Part model, mm, in its own coordinate system. Round coordinates to 2 decimals unless told otherwise and drop trailing zeros. Order: outer loops, then holes, each group sorted by start corner. A loop starts at its lowest first (then second) coordinate and runs counter-clockwise, first axis right, second up. Notation, with made-up numbers: (74.5, 49.25) - (128.5, 49.25) arc R36 cw to (128.5, 88.25) - close; hole circle Ø11 at (-35, -23.5). An arc over 180 degrees is marked (long way). Answer as a JSON object with one key per item and string values.
```python
from build123d import *

# Parameters (mm, degrees)
SKETCH1_R           = 254.5
SKETCH1_R_2         = 234.5
BOSS_EXTRUDE1_DEPTH = 5
SKETCH2_W           = 27.805822748
SKETCH2_H           = 60
CUT_EXTRUDE1_DEPTH  = 5
SKETCH3_R           = 2.5
CUT_EXTRUDE2_DEPTH  = 5
SKETCH4_R           = 1.5
CUT_EXTRUDE3_DEPTH  = 5


with BuildPart() as part:
    # Sketch1 → Boss-Extrude1 (new body)
    with BuildSketch(Plane(origin=(0, 0, 0), x_dir=(1, 0, 0), z_dir=(0, 1, 0))):
        with Locations(Location((0, 0, 0), (0, 0, 270))):
            Circle(SKETCH1_R)
        with Locations(Location((0, 0, 0), (0, 0, 270))):
            Circle(SKETCH1_R_2, mode=Mode.SUBTRACT)
    extrude(amount=BOSS_EXTRUDE1_DEPTH)

    # Sketch2 → Cut-Extrude1 (cut)
    with BuildSketch(Plane(origin=(0, 5, 0), x_dir=(1, 0, 0), z_dir=(0, 1, 0))):
        with Locations((-240.597088626, 30)):
            Rectangle(SKETCH2_W, SKETCH2_H)
    cut_extrude1 = extrude(amount=-CUT_EXTRUDE1_DEPTH, mode=Mode.SUBTRACT)

    # Mirror1: Cut-Extrude1 across plane
    add(cut_extrude1.mirror(Plane.XY), mode=Mode.SUBTRACT)

    # Sketch3 → Cut-Extrude2 (cut)
    with BuildSketch(Plane(origin=(0, 5, 0), x_dir=(1, 0, 0), z_dir=(0, 1, 0))):
        with Locations(Location((242.5, 0, 0), (0, 0, 270))):
            Circle(SKETCH3_R)
        with Locations(Location((196.186621136, -142.537923681, 0), (0, 0, 270))):
            Circle(SKETCH3_R)
        with Locations(Location((74.936621136, -230.631205202, 0), (0, 0, 270))):
            Circle(SKETCH3_R)
        with Locations(Location((-74.936621136, -230.631205202, 0), (0, 0, 270))):
            Circle(SKETCH3_R)
        with Locations(Location((-196.186621136, -142.537923681, 0), (0, 0, 270))):
            Circle(SKETCH3_R)
        with Locations((-242.5, 0)):
            Circle(SKETCH3_R)
        with Locations(Location((-196.186621136, 142.537923681, 0), (0, 0, 270))):
            Circle(SKETCH3_R)
        with Locations(Location((-74.936621136, 230.631205202, 0), (0, 0, 270))):
            Circle(SKETCH3_R)
        with Locations(Location((74.936621136, 230.631205202, 0), (0, 0, 270))):
            Circle(SKETCH3_R)
        with Locations(Location((196.186621136, 142.537923681, 0), (0, 0, 270))):
            Circle(SKETCH3_R)
    extrude(amount=-CUT_EXTRUDE2_DEPTH, mode=Mode.SUBTRACT)

    # Sketch4 → Cut-Extrude3 (cut)
    with BuildSketch(Plane(origin=(0, 5, 0), x_dir=(1, 0, 0), z_dir=(0, 1, 0))):
        with Locations(Location((0, -242.5, 0), (0, 0, 270))):
            Circle(SKETCH4_R)
        with Locations(Location((-142.537923681, -196.186621136, 0), (0, 0, 270))):
            Circle(SKETCH4_R)
        with Locations(Location((-230.631205202, -74.936621136, 0), (0, 0, 270))):
            Circle(SKETCH4_R)
        with Locations(Location((-230.631205202, 74.936621136, 0), (0, 0, 270))):
            Circle(SKETCH4_R)
        with Locations(Location((-142.537923681, 196.186621136, 0), (0, 0, 270))):
            Circle(SKETCH4_R)
        with Locations(Location((0, 242.5, 0), (0, 0, 270))):
            Circle(SKETCH4_R)
        with Locations(Location((142.537923681, 196.186621136, 0), (0, 0, 270))):
            Circle(SKETCH4_R)
        with Locations(Location((230.631205202, 74.936621136, 0), (0, 0, 270))):
            Circle(SKETCH4_R)
        with Locations(Location((230.631205202, -74.936621136, 0), (0, 0, 270))):
            Circle(SKETCH4_R)
        with Locations(Location((142.537923681, -196.186621136, 0), (0, 0, 270))):
            Circle(SKETCH4_R)
    extrude(amount=-CUT_EXTRUDE3_DEPTH, mode=Mode.SUBTRACT)


solid = part.part
```
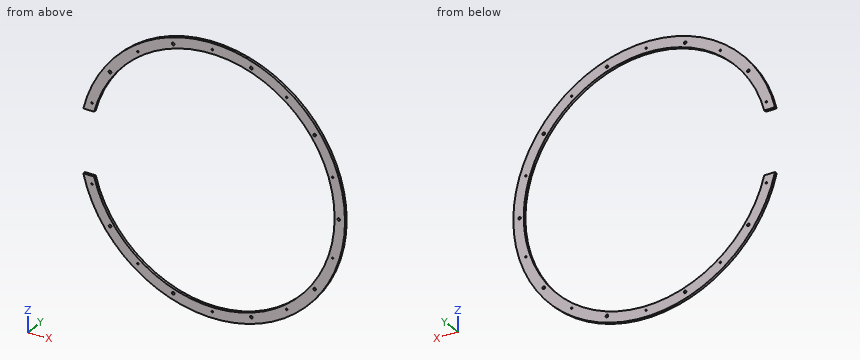
Item 1: Cut at B-B (x = 97). Write the cut outline in (y, z), plus the area to 3 significant figures.
Taken from the geometry:
{"outline": "(0, -235.29) - (5, -235.29) - (5, -213.5) - (0, -213.5) - close; (0, 213.5) - (5, 213.5) - (5, 235.29) - (0, 235.29) - close", "area": "218 mm2"}
Item 2: Cut at D-D (z = 33.5). Write the cut outline in (x, y), plus the area to 3 significant figures.
Taken from the geometry:
{"outline": "(232.09, 0) - (252.29, 0) - (252.29, 5) - (232.09, 5) - close", "area": "101 mm2"}
Item 3: Probe L1, parallel to Z at x = 1, y = 2.45; L2, parallel to X at y = 3.2, z = -5.5; L3, parallel to Z at x = 142, y = 0.75. List the from-to ranges inside material, lowest first. Write a range as from..to.
Taken from the geometry:
{"L1": "-254.5..-243.62, -241.38..-234.5, 234.5..241.38, 243.62..254.5", "L2": "234.44..254.44", "L3": "-211.2..-197.59, -194.79..-186.62, 186.62..194.79, 197.59..211.2"}
Item 4: Drop flat-ended pins along their axis: P1, Ø2.5, axis at x = -230.63, z = 74.94, coming from the +Y side; P2, Ø1, axis at y = 2, z = -199, coming from the -X side; P3, Ø2.5, axis at x = -236.5, y = 2, coming from the -Z side. Give the stop position or say it passes through.
Taken from the geometry:
{"P1": "through", "P2": "x = -159.27", "P3": "z = -97.1"}
Item 5: Cut at A-A (z = -124). Write the cut outline in (x, y), plus the area to 3 significant figures.
Taken from the geometry:
{"outline": "(-222.25, 0) - (-199.03, 0) - (-199.03, 5) - (-222.25, 5) - close; (199.03, 0) - (222.25, 0) - (222.25, 5) - (199.03, 5) - close", "area": "232 mm2"}
Item 6: Cut at C-C (y = 3.25). State how many separate pieces and enclosed holes the cut face has, plus the area to 3 significant figures.
Taken from the geometry:
{"separate pieces": "1", "enclosed holes": "19", "area": "28,100 mm2"}
